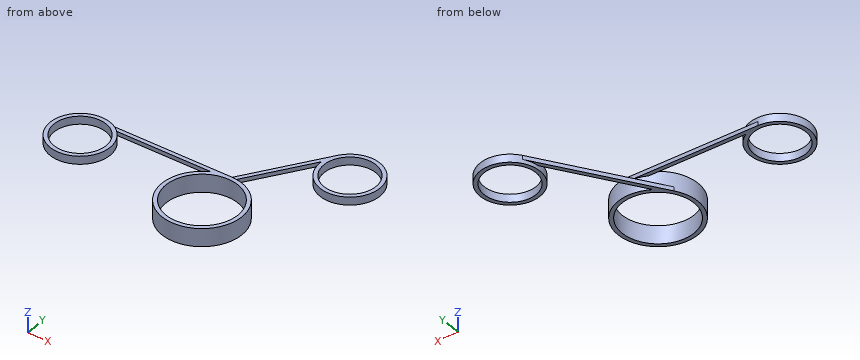
```python
from build123d import *

# Parameters (mm, degrees)
SKETCH1_R           = 10
BOSS_EXTRUDE1_DEPTH = 4.5
SKETCH2_R           = 9
CUT_EXTRUDE1_DEPTH  = 4.5
SKETCH3_W           = 32.5
SKETCH3_H           = 1
BOSS_EXTRUDE2_DEPTH = 1
SKETCH5_R           = 7.5
BOSS_EXTRUDE3_DEPTH = 1
SKETCH6_R           = 6.5
CUT_EXTRUDE2_DEPTH  = 2
BOSS_EXTRUDE4_DEPTH = 1
SKETCH9_R           = 7.5
BOSS_EXTRUDE5_DEPTH = 1
SKETCH10_R          = 6.5
CUT_EXTRUDE3_DEPTH  = 2


with BuildPart() as part:
    # Sketch1 → Boss-Extrude1 (new body)
    with BuildSketch(Plane.XY):
        Circle(SKETCH1_R)
    extrude(amount=BOSS_EXTRUDE1_DEPTH)

    # Sketch2 → Cut-Extrude1 (cut)
    with BuildSketch(Plane.XY.offset(4.5)):
        Circle(SKETCH2_R)
    extrude(amount=-CUT_EXTRUDE1_DEPTH, mode=Mode.SUBTRACT)

    # Sketch3 → Boss-Extrude2 (add)
    with BuildSketch(Plane.XY.offset(4.5)):
        with Locations((-16.25, 9.5)):
            Rectangle(SKETCH3_W, SKETCH3_H)
    extrude(amount=-BOSS_EXTRUDE2_DEPTH)

    # Sketch5 → Boss-Extrude3 (add, symmetric)
    with BuildSketch(Plane.XY.offset(4.5)):
        with Locations((-32.5, 2.5)):
            Circle(SKETCH5_R)
    extrude(amount=BOSS_EXTRUDE3_DEPTH, both=True)

    # Sketch6 → Cut-Extrude2 (cut)
    with BuildSketch(Plane.XY.offset(5.5)):
        with Locations((-32.5, 2.5)):
            Circle(SKETCH6_R)
    extrude(amount=-CUT_EXTRUDE2_DEPTH, mode=Mode.SUBTRACT)

    # Sketch8 → Boss-Extrude4 (add)
    with BuildSketch(Plane(origin=(0, 0, 0), x_dir=(-1, 0, 0), z_dir=(0, 0, -1))):
        Polygon((8.194096935, 5.732082992), (-9.885510569, 32.739078243), (-10.716495038, 32.182782628), (7.362918515, 5.175657537), align=None)
    extrude(amount=-BOSS_EXTRUDE4_DEPTH)

    # Sketch9 → Boss-Extrude5 (add, symmetric)
    with BuildSketch(Plane(origin=(0, 0, 0), x_dir=(-1, 0, 0), z_dir=(0, 0, -1))):
        with Locations((-16.117894088, 28.566861127)):
            Circle(SKETCH9_R)
    extrude(amount=BOSS_EXTRUDE5_DEPTH, both=True)

    # Sketch10 → Cut-Extrude3 (cut)
    with BuildSketch(Plane(origin=(0, 0, -1), x_dir=(-1, 0, 0), z_dir=(0, 0, -1))):
        with Locations((-16.117894088, 28.566861127)):
            Circle(SKETCH10_R)
    extrude(amount=-CUT_EXTRUDE3_DEPTH, mode=Mode.SUBTRACT)


solid = part.part
```
Source: CAD feature listing. Evaluate the final solid. Frame: model axes, mm. Coordinates: 2 decimals unless noted, no trailing zeros. Write each loop counter-clockwise with the first axis right and the second up, starting at its lowest first coordinate (ties: lowest second). Pieces come first, ordered by that corner, then holes. Notation, with made-up numbers: (40.25, -31.75) - (85.25, -31.75) arc R10 cw to (85.25, -19.75) - close; hole circle Ø7 at (34, 48.25). An arc over 180 degrees is marked (long way). Answer as a JSON object with one key per item and string values.
Q1. First-contact query: pin 1 Ø3 at (x, z) = (-30.5, 1.5) entering from -Y; pin 2 Ø17 at (x, y) = (-32.5, 2.5) entering from -Z; pin 3 Ø10 at (x, y) = (2, 15) entering from -Z; pin 4 Ø6 at (x, y) = (-8.5, -4.5) entering from +Z. Flat tips, straight axial feed; report the tip coordinate or a pass-through.
Ans:
{"pin 1": "passes through", "pin 2": "stops at z = 3.5", "pin 3": "stops at z = 0", "pin 4": "stops at z = 4.5"}
Q2. Section query C-C, the plane y = 23.5. Output: boundary loops of the cut face in (x, z).
Ans:
{"outline": "(3.7, 0) - (4.9, 0) - (4.9, 1) - (3.7, 1) - close; (10.59, -1) - (12.05, -1) - (12.05, 1) - (10.59, 1) - close; (20.19, -1) - (21.65, -1) - (21.65, 1) - (20.19, 1) - close"}
Q3. Section query B-B, the plane y = -6. Output: boundary loops of the cut face in (x, z).
Ans:
{"outline": "(-8, 0) - (-6.71, 0) - (-6.71, 4.5) - (-8, 4.5) - close; (6.71, 0) - (8, 0) - (8, 4.5) - (6.71, 4.5) - close"}
Q4. Section query A-A, the plane y = 2.5. Output: boundary loops of the cut face in (x, z).
Ans:
{"outline": "(-40, 3.5) - (-39, 3.5) - (-39, 5.5) - (-40, 5.5) - close; (-26, 3.5) - (-25, 3.5) - (-25, 5.5) - (-26, 5.5) - close; (-9.68, 0) - (-8.65, 0) - (-8.65, 4.5) - (-9.68, 4.5) - close; (8.65, 0) - (9.68, 0) - (9.68, 4.5) - (8.65, 4.5) - close"}
Q5. Material intervals for line 1 (Y direction, x = 0, z = 1.25); line 2 (Y direction, x = -32.5, z = 5.1), sorted ascending. Write a range as [from, to].
Ans:
{"line 1": "y = [-10, -9], [9, 10]", "line 2": "y = [-5, -4], [9, 10]"}
Q6. Section query D-D, the plane x = 3.5. Output: boundary loops of the cut face in (y, z), plus the area to 3 significant figures.
Ans:
{"outline": "(-9.37, 0) - (-8.29, 0) - (-8.29, 4.5) - (-9.37, 4.5) - close; (8.29, 0) - (9.37, 0) - (9.37, 4.5) - (8.29, 4.5) - close; (21.4, 0) - (23.2, 0) - (23.2, 1) - (21.4, 1) - close", "area": "11.5 mm2"}
